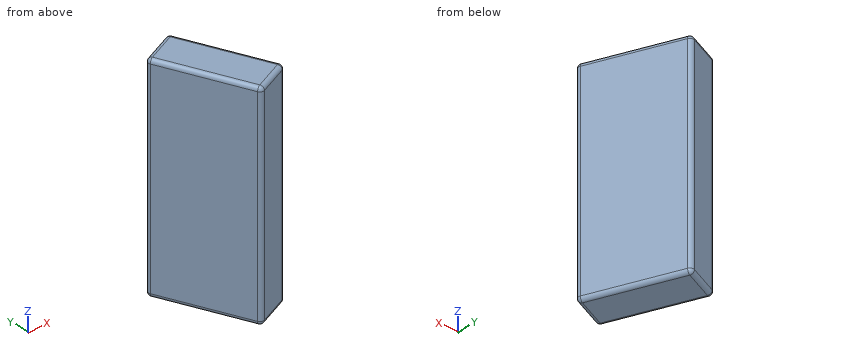
from build123d import *

# Parameters (mm, degrees)
F2_DEPTH = 5.5
F4_R     = 0.2


with BuildPart() as f2:
    # F1 (on Top) → F2 (new body)
    with BuildSketch(Plane.XY):
        Polygon((24.6480524192, 21.7062796455), (22.8097623591, 20.9184410483), (24.779358852, 16.3227158982), (26.617648912, 17.1105544954), align=None)
    extrude(amount=F2_DEPTH)

    # F3: F2 across plane


with BuildPart() as f2_1:
    add(f2.part)
    add(f2.part.mirror(Plane.XY))

    # F4
    f4_edges = [f2_1.edges().sort_by_distance(p)[0] for p in [
        (25.698504, 16.716635, 5.5),
        (26.617649, 17.110554, 0),
        (25.698504, 16.716635, -5.5),
        (24.779359, 16.322716, 0),
        (23.794561, 18.620578, 5.5),
        (25.632851, 19.408417, 5.5),
        (23.728907, 21.31236, 5.5),
        (24.648052, 21.70628, 0),
        (22.809762, 20.918441, 0),
        (23.728907, 21.31236, -5.5),
        (23.794561, 18.620578, -5.5),
        (25.632851, 19.408417, -5.5),
    ]]
    fillet(f4_edges, radius=F4_R)


solid = f2_1.part
Build history of the part. All positions in model axes, mm. Coordinates: 2 decimals unless noted, no trailing zeros. Order: outer loops, then holes, each group sorted by start corner. A loop starts at its lowest first (then second) coordinate and runs counter-clockwise, first axis right, second up. Notation, with made-up numbers: (59.25, 45.5) - (63.25, 45.5) arc R37 cw to (63.25, 81.5) - close; hole circle Ø10 at (69.5, 55.5). An arc over 180 degrees is marked (long way). Put each result on its own line as item: value.
1. Probe line 1 along X through (y, z) = (20.25, 0.5); line 2 along X through (y, z) = (20.1, -4); line 3 along Y through (x, z) = (24.55, -1.75). List the from-to ranges inside material, lowest first. Write a range as [from, to].
Answer sheet:
line 1: x = [23.1, 25.27]
line 2: x = [23.16, 25.34]
line 3: y = [16.86, 21.64]
2. Saw through at A-A (z = -2). Write the cut outline in (x, y).
Answer sheet:
outline: (22.89, 20.73) - (24.7, 16.51) arc R0.2 ccw to (24.96, 16.4) - (26.43, 17.03) arc R0.2 ccw to (26.54, 17.29) - (24.73, 21.52) arc R0.2 ccw to (24.46, 21.63) - (22.99, 21) arc R0.2 ccw to start
3. Drop flat-ended pins along their axis: P1, Ø3, axis at y = 20, z = 3, coming from the +X side; P2, Ø2, axis at y = 20.5, z = 1.5, coming from the +X side. Give the stop position or say it passes through.
Answer sheet:
P1: stops at x = 26.02
P2: stops at x = 25.59
